Part model, mm, in its own coordinate system. Give positions to 0.01 mm unless a question says otherwise; leave off trailing zeros. Order: outer loops, then holes, each group sorted by start corner. A loop starts at its lowest first (then second) coordinate and runs counter-clockwise, first axis right, second up. Notation, with made-up numbers: (70, 28.5) -> (75, 28.5) arc R14 ccw to (75, 38.5) -> close; hole circle Ø5 at (71, 1.5). An arc over 180 degrees is marked (long way). Write item = value, one per line. Start each with the question number.
Item 1: Band-saw the part on A-A on z = -42.25. Write the cut outline in (x, y), plus the area to 3 significant figures.
Item 2: Band-saw the part on B-B on x = -94.25. Write the cut outline in (y, z), plus the area to 3 significant figures.
Item 3: Drill centre lines: line 1 along X through (y, z) = (84.45, -53.75); line 2 along Z through (x, y) = (-84, 84.5); line 3 along X through (y, z) = (84.5, -42.5). Where is each one in solid material? Low to high.
Item 4: Band-saw the part on D-D on z = -50.5. Write the cut outline in (x, y).
Item 5: Band-saw the part on C-C on y = 84.25. Write the cut outline in (x, z) (3 decimals).
Item 6: Pull direction Z, two halves, no side cores. Call faces 1 (the face through (-89, 85.08, -47)), 2 (the face through (-81.51, 84.59, -53.05)), 3 (the face through (-78.448, 84.587, -54.032)): +Z half, -Z half, draft (parallel to the pull), parting line (faces both ways), or undercut.
Item 7: Flat gauge pin, fed straight in: P1, Ø2.5, axis at x = -95.07, z = -41.26, coming from the +Y side. Where does the tip first touch, or does it go through?
```python
from build123d import *

# Parameters (mm, degrees)
SKETCH1_R           = 12.6
SKETCH1_R_2         = 1.575
BOSS_EXTRUDE1_DEPTH = 1


with BuildPart() as part:
    # Sketch1 → Boss-Extrude1 (new body)
    with BuildSketch(Plane.XZ.offset(-85.080072415)):
        with Locations(Location((-89.072792821, -47.25870832, 0), (0, 0, 270))):
            Circle(SKETCH1_R)
        with Locations(Location((-95.072792821, -41.25870832, 0), (0, 0, 270))):
            Circle(SKETCH1_R_2, mode=Mode.SUBTRACT)
        with Locations(Location((-83.072792821, -41.25870832, 0), (0, 0, 270))):
            Circle(SKETCH1_R_2, mode=Mode.SUBTRACT)
        with Locations(Location((-83.072792821, -53.25870832, 0), (0, 0, 270))):
            Circle(SKETCH1_R_2, mode=Mode.SUBTRACT)
        with Locations(Location((-95.072792821, -53.25870832, 0), (0, 0, 270))):
            Circle(SKETCH1_R_2, mode=Mode.SUBTRACT)
    extrude(amount=BOSS_EXTRUDE1_DEPTH)


solid = part.part
```
Values found:
q1.outline = (-100.63, 84.08) -> (-96.3, 84.08) -> (-96.3, 85.08) -> (-100.63, 85.08) -> close; (-93.85, 84.08) -> (-84.3, 84.08) -> (-84.3, 85.08) -> (-93.85, 85.08) -> close; (-81.85, 84.08) -> (-77.51, 84.08) -> (-77.51, 85.08) -> (-81.85, 85.08) -> close
q1.area = 18.2 mm^2
q2.outline = (84.08, -58.75) -> (85.08, -58.75) -> (85.08, -54.6) -> (84.08, -54.6) -> close; (84.08, -51.92) -> (85.08, -51.92) -> (85.08, -42.6) -> (84.08, -42.6) -> close; (84.08, -39.92) -> (85.08, -39.92) -> (85.08, -35.77) -> (84.08, -35.77) -> close
q2.area = 17.6 mm^2
q3.line_1 = -99.87 to -96.57, -93.58 to -84.57, -81.58 to -78.27
q3.line_2 = -58.79 to -54.53, -51.99 to -42.53, -39.99 to -35.72
q3.line_3 = -100.74 to -96.04, -94.1 to -84.04, -82.1 to -77.41
q4.outline = (-101.25, 84.08) -> (-76.9, 84.08) -> (-76.9, 85.08) -> (-101.25, 85.08) -> close
q5.outline = circle Ø25.2 at (-89.073, -47.259); hole circle Ø3.15 at (-95.073, -53.259); hole circle Ø3.15 at (-95.073, -41.259); hole circle Ø3.15 at (-83.073, -53.259); hole circle Ø3.15 at (-83.073, -41.259)
q6.face_1 = draft
q6.face_2 = undercut
q6.face_3 = parting line
q7.P1 = through
